Build history of the part. All positions in model axes, mm. Face numbers are marked on the shaded views. A direction names the side the tool comes from. Coordinates: 2 decimals unless noted, no trailing zeros. Loops run counter-clockwise (first coordinate to the right, second up) from the corner with the lowest first, then second, coordinate; pieces in that order, holes last. Notation, with made-up numbers: (88.25, 61.25) - (124.25, 61.25) arc R24 ccw to (124.25, 83.25) - close; hole circle Ø6 at (33.25, 74). An arc over 180 degrees is marked (long way). One line per item, written item: value.
```python
from build123d import *

# Parameters (mm, degrees)
F0_R     = 14.2875
F1_DEPTH = 25.4
F2_DEPTH = 50.8
F3_R     = 14.2875
F4_DEPTH = 50.8


with BuildPart() as f1:
    # F0 (on Front) → F1 (new body)
    with BuildSketch(Plane.XZ):
        with BuildLine():
            ThreePointArc((5.0426470588, -28.1265414802), (21.9160245563, -18.3362616868), (28.575, 0))
            ThreePointArc((28.575, 0), (21.9160245563, 18.3362616868), (5.0426470588, 28.1265414802))
            ThreePointArc((5.0426470588, 28.1265414802), (-28.575, 0), (5.0426470588, -28.1265414802))
        make_face()
        with BuildLine():
            ThreePointArc((-13.4703841816, 4.7625), (0, 14.2875), (13.4703841816, 4.7625))
            Line((13.4703841816, 4.7625), (19.05, 4.7625))
            Line((19.05, 4.7625), (19.05, -4.7625))
            Line((19.05, -4.7625), (13.4703841816, -4.7625))
            ThreePointArc((13.4703841816, -4.7625), (0, -14.2875), (-13.4703841816, -4.7625))
            Line((-13.4703841816, -4.7625), (-19.05, -4.7625))
            Line((-19.05, -4.7625), (-19.05, 4.7625))
            Line((-19.05, 4.7625), (-13.4703841816, 4.7625))
        make_face(mode=Mode.SUBTRACT)
        with BuildLine():
            ThreePointArc((-13.4703841816, -4.7625), (-14.2875, 0), (-13.4703841816, 4.7625))
            Line((-13.4703841816, 4.7625), (-19.05, 4.7625))
            Line((-19.05, 4.7625), (-19.05, -4.7625))
            Line((-19.05, -4.7625), (-13.4703841816, -4.7625))
        make_face()
        with BuildLine():
            ThreePointArc((5.0426470588, 28.1265414802), (21.9160245563, 18.3362616868), (28.575, 0))
            ThreePointArc((28.575, 0), (21.9160245563, -18.3362616868), (5.0426470588, -28.1265414802))
            Line((5.0426470588, -28.1265414802), (57.3367647059, -18.7510276535))
            ThreePointArc((57.3367647059, -18.7510276535), (34.925, 0), (57.3367647059, 18.7510276535))
            Line((57.3367647059, 18.7510276535), (5.0426470588, 28.1265414802))
        make_face()
        with BuildLine():
            ThreePointArc((73.025, 0), (68.5856830375, 12.2241744579), (57.3367647059, 18.7510276535))
            ThreePointArc((57.3367647059, 18.7510276535), (34.925, 0), (57.3367647059, -18.7510276535))
            ThreePointArc((57.3367647059, -18.7510276535), (68.5856830375, -12.2241744579), (73.025, 0))
        make_face()
        with Locations((53.975, 0)):
            Circle(F0_R, mode=Mode.SUBTRACT)
    extrude(amount=F1_DEPTH)

    # F0 (on Front) → F2 (join)
    with BuildSketch(Plane.XZ):
        with BuildLine():
            ThreePointArc((5.0426470588, -28.1265414802), (21.9160245563, -18.3362616868), (28.575, 0))
            ThreePointArc((28.575, 0), (21.9160245563, 18.3362616868), (5.0426470588, 28.1265414802))
            ThreePointArc((5.0426470588, 28.1265414802), (-28.575, 0), (5.0426470588, -28.1265414802))
        make_face()
        with BuildLine():
            ThreePointArc((-13.4703841816, 4.7625), (0, 14.2875), (13.4703841816, 4.7625))
            Line((13.4703841816, 4.7625), (19.05, 4.7625))
            Line((19.05, 4.7625), (19.05, -4.7625))
            Line((19.05, -4.7625), (13.4703841816, -4.7625))
            ThreePointArc((13.4703841816, -4.7625), (0, -14.2875), (-13.4703841816, -4.7625))
            Line((-13.4703841816, -4.7625), (-19.05, -4.7625))
            Line((-19.05, -4.7625), (-19.05, 4.7625))
            Line((-19.05, 4.7625), (-13.4703841816, 4.7625))
        make_face(mode=Mode.SUBTRACT)
        with BuildLine():
            ThreePointArc((-13.4703841816, -4.7625), (-14.2875, 0), (-13.4703841816, 4.7625))
            Line((-13.4703841816, 4.7625), (-19.05, 4.7625))
            Line((-19.05, 4.7625), (-19.05, -4.7625))
            Line((-19.05, -4.7625), (-13.4703841816, -4.7625))
        make_face()
    extrude(amount=F2_DEPTH)

    # F3 (on face) → F4 (join, through all)
    with BuildSketch(Plane.XZ.offset(50.8)):
        with BuildLine():
            Line((-28.575, 60.9835536748), (-28.575, 0))
            ThreePointArc((-28.575, 0), (0, 28.575), (28.575, 0))
            Line((28.575, 0), (28.575, 67.3335536748))
            Line((28.575, 67.3335536748), (-22.225, 67.3335536748))
            ThreePointArc((-22.225, 67.3335536748), (-26.7151280605, 65.4736817353), (-28.575, 60.9835536748))
        make_face()
        with Locations((53.975, 0)):
            Circle(F3_R)
    extrude(amount=-F4_DEPTH)


solid = f1.part
```
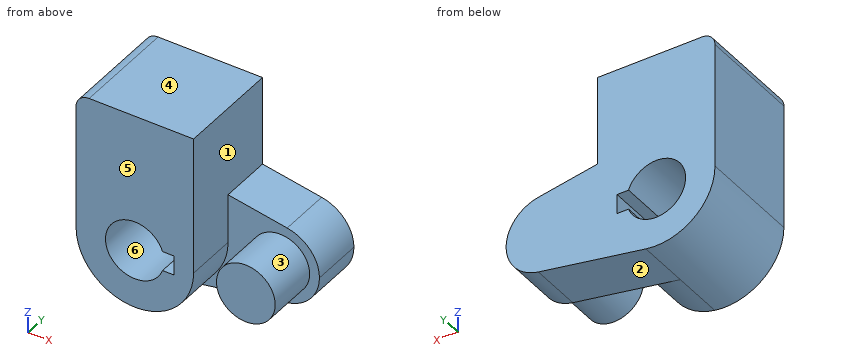
Item 1: Tool access for the marked faces 1, 2 and 3: list every direction of +Z, -Z, +X, -X, +Y, -Y with a clear straight run to the whole face (end or side of a thin tool).
Check result:
face 1: +Z, -Y
face 2: -Z, +X, +Y, -Y
face 3: -Y
Item 2: Cut at B-B, the plane x = 0. Write the cut outline in (y, z) (1 decimal), then the cut area to 3 significant figures.
Check result:
outline: (-50.8, -28.6) - (0, -28.6) - (0, -14.3) - (-50.8, -14.3) - close; (-50.8, 14.3) - (0, 14.3) - (0, 67.3) - (-50.8, 67.3) - close
area: 3,420 mm^2
Item 3: Drop flat-ended pins along their axis: P1, Ø4, axis at x = 48, y = -28.5, coming from the +Z side; P2, Ø10, axis at y = -45, z = -9, coming from the +X side; P3, Ø12, axis at x = 12, y = -5, coming from the -Z side. Give the stop position or say it passes through.
Check result:
P1: stops at z = 13.72
P2: stops at x = 67.69
P3: stops at z = -27.95
Item 4: Pull direction Z, two halves, no side cores. Call the marked faces 4, 5 and 6: released by +Z, released by -Z, zero draft, split by the parting line, or undercut.
Check result:
face 4: released by +Z
face 5: zero draft
face 6: undercut
Item 5: Cut at D-D, the plane z = 11. Write the cut outline in (x, y) (3 decimals), then the cut area to 3 significant figures.
Check result:
outline: (-28.575, -50.8) - (-9.118, -50.8) - (-9.118, 0) - (-28.575, 0) - close; (9.118, -50.8) - (28.575, -50.8) - (28.575, -25.4) - (44.857, -25.4) - (44.857, -50.8) - (63.093, -50.8) - (63.093, -25.4) - (69.528, -25.4) - (69.528, 0) - (9.118, 0) - close
area: 3,480 mm^2
Item 6: Probe probe 1 along Z at (x, y) = (0, -19.5) (1 decimal); probe 2 along Z at (x, y) = (-2, -23.5); probe 3 along X at (y, z) = (-15.5, 55.5) (3 decimals). List the from-to ranges inside material, lowest first. Write a range as from..to.
Check result:
probe 1: z = -28.6..-14.3, 14.3..67.3
probe 2: z = -28.5..-14.15, 14.15..67.33
probe 3: x = -28.575..28.575
Item 7: Cut at A-A, the plane y = -30.5. Give the number of separate pieces and of enclosed holes in the cut face, then the cut area to 3 significant figures.
Check result:
separate pieces: 2
enclosed holes: 1
area: 5,070 mm^2
